Verification items for the finished model (mm, model axes). A direction names the side the tool comes from. Coordinates: 2 decimals unless noted, no trailing zeros. Order: outer loops, then holes, each group sorted by start corner. A loop starts at its lowest first (then second) coordinate and runs counter-clockwise, first axis right, second up. Notation, with made-up numbers: M 4.5,35 L 41.5,35 A15 cw 41.5,53 Z; hole C 2,-9.75 d3. An arc over 180 degrees is marked long. Return JSON: item names as keys, results as strings. Group by question number.
Q1. Section check A-A, the plane x = -34. Enter the section's corners in (y, z).
Q2. Go/stop test with flat-tipped pins: pin 1 Ø3 at (y, z) = (-21, 4) entering from -X; pin 2 Ø3 at (x, z) = (26.5, 3.5) entering from +Y; pin 3 Ø1 at (x, y) = (12, 22) entering from +Z; pin 4 Ø1.5 at (x, z) = (17, -2.5) entering from -Y. Record where each tip stops, or that it passes through.
Q3. Mould release check, pull along Y, two halves, no side actions. Record for faces 5 (the face through (-27, -23, 3)), 6 (the face through (19.772, 23.235, 3.965)), 7 (the face through (-35.11, 21.01, 0.76)), 8 (the face through (-0.8, -20, 3)): pulls with the +Y half, pulls with the -Y half, needs draft (parallel to the pull), parting line crosses it, or undercut.
Q4. Section check C-C, the plane x = 27.5. Enter the section's corners in (y, z), then the cut area to 3 significant figures.
Q5. Thickness scan on probe 1 along Y at (x, z) = (34, 0.55); probe 2 along Y at (x, z) = (-12, 2.25); probe 3 along Z at (x, y) = (-17, 8). Record the ranges inside material, lowest first.
Q6. Section check D-D, the plane z = -8. Enter the section's corners in (x, y), then the cut area to 3 significant figures.
Q7. Section check B-B, the plane y = 10. Enter the section's corners in (x, z), then the cut area to 3 significant figures.
Q8. Access from +Z, -Z, +X, -X, +Y, -Y to the whole of each face (thin tool, end or side, straight path). Record for faces 1 (the face through (-32, -7, -5)), 2 (the face through (-28, -21.3, 5.5)), 3 (the face through (-20, 22, 6.5)), 4 (the face through (27, -20, 7)).
from build123d import *

# Parameters (mm, degrees)
SKETCH_W     = 76
SKETCH_H     = 50
PAD_DEPTH    = 1.5
SKETCH001_R  = 1.5
POCKET_DEPTH = 1.501
SKETCH002_R  = 1.75
PAD001_DEPTH = 5
SKETCH003_W  = 61
SKETCH003_H  = 14
PAD002_DEPTH = 7
SKETCH004_W  = 6
SKETCH004_H  = 15
PAD003_DEPTH = 10
SKETCH005_W  = 6
SKETCH005_H  = 6
PAD004_DEPTH = 4
SKETCH006_R  = 1.75
PAD005_DEPTH = 1.5


with BuildPart() as part:
    # Sketch → Pad (new body)
    with BuildSketch(Plane.XY):
        Rectangle(SKETCH_W, SKETCH_H)
    extrude(amount=PAD_DEPTH)

    # Sketch001 (on Face6 of Pad) → Pocket (cut, through all)
    with BuildSketch(Plane.XY.offset(1.5)):
        with Locations((-34, 20)):
            Circle(SKETCH001_R)
        with Locations((34, 20)):
            Circle(SKETCH001_R)
        with Locations((-34, -20)):
            Circle(SKETCH001_R)
        with Locations((34, -20)):
            Circle(SKETCH001_R)
    extrude(amount=-POCKET_DEPTH, mode=Mode.SUBTRACT)

    # Sketch002 (on Face5 of Pocket) → Pad001 (join)
    with BuildSketch(Plane.XY.offset(1.5)):
        with Locations((-28, 21.5)):
            Circle(SKETCH002_R)
        with Locations((-20, 21.5)):
            Circle(SKETCH002_R)
        with Locations((-12, 21.5)):
            Circle(SKETCH002_R)
        with Locations((-4, 21.5)):
            Circle(SKETCH002_R)
        with Locations((4, 21.5)):
            Circle(SKETCH002_R)
        with Locations((12, 21.5)):
            Circle(SKETCH002_R)
        with Locations((20, 21.5)):
            Circle(SKETCH002_R)
        with Locations((28, 21.5)):
            Circle(SKETCH002_R)
    extrude(amount=PAD001_DEPTH)

    # Sketch003 (on Face5 of Pad001) → Pad002 (join)
    with BuildSketch(Plane.XY.offset(1.5)):
        with Locations((0, 9)):
            Rectangle(SKETCH003_W, SKETCH003_H)
    extrude(amount=PAD002_DEPTH)

    # Sketch004 (on Face4 of Pad002) → Pad003 (join)
    with BuildSketch(Plane(origin=(0, 0, 0), x_dir=(1, 0, 0), z_dir=(0, 0, -1))):
        with Locations((-35, 7.5)):
            Rectangle(SKETCH004_W, SKETCH004_H)
    extrude(amount=PAD003_DEPTH)

    # Sketch005 (on Face5 of Pad003) → Pad004 (join)
    with BuildSketch(Plane.XY.offset(1.5)):
        with Locations((-26.6, -20)):
            Rectangle(SKETCH005_W, SKETCH005_H)
        with Locations((-19, -20)):
            Rectangle(SKETCH005_W, SKETCH005_H)
        with Locations((-11.4, -20)):
            Rectangle(SKETCH005_W, SKETCH005_H)
        with Locations((-3.8, -20)):
            Rectangle(SKETCH005_W, SKETCH005_H)
        with Locations((3.8, -20)):
            Rectangle(SKETCH005_W, SKETCH005_H)
        with Locations((11.4, -20)):
            Rectangle(SKETCH005_W, SKETCH005_H)
        with Locations((19, -20)):
            Rectangle(SKETCH005_W, SKETCH005_H)
        with Locations((26.6, -20)):
            Rectangle(SKETCH005_W, SKETCH005_H)
    extrude(amount=PAD004_DEPTH)

    # Sketch006 (on Face67 of Pad004) → Pad005 (join)
    with BuildSketch(Plane.XY.offset(5.5)):
        with Locations((-26.6, -20)):
            Circle(SKETCH006_R)
        with Locations((-19, -20)):
            Circle(SKETCH006_R)
        with Locations((-11.4, -20)):
            Circle(SKETCH006_R)
        with Locations((-3.8, -20)):
            Circle(SKETCH006_R)
        with Locations((3.8, -20)):
            Circle(SKETCH006_R)
        with Locations((11.4, -20)):
            Circle(SKETCH006_R)
        with Locations((19, -20)):
            Circle(SKETCH006_R)
        with Locations((26.6, -20)):
            Circle(SKETCH006_R)
    extrude(amount=PAD005_DEPTH)


solid = part.part
Numbers:
{
 "1": {"outline": "M -25,0 L -21.5,0 L -21.5,1.5 L -25,1.5 Z; M -18.5,0 L -15,0 L -15,-10 L 0,-10 L 0,0 L 18.5,0 L 18.5,1.5 L -18.5,1.5 Z; M 21.5,0 L 25,0 L 25,1.5 L 21.5,1.5 Z"},
 "2": {"pin 1": "stops at x = -29.6", "pin 2": "stops at y = 23.25", "pin 3": "stops at z = 6.5", "pin 4": "passes through"},
 "3": {"face 5": "pulls with the -Y half", "face 6": "undercut", "face 7": "undercut", "face 8": "needs draft"},
 "4": {"outline": "M -25,0 L 25,0 L 25,1.5 L 23.18,1.5 L 23.18,6.5 L 19.82,6.5 L 19.82,1.5 L 16,1.5 L 16,8.5 L 2,8.5 L 2,1.5 L -17,1.5 L -17,5.5 L -18.5,5.5 L -18.5,7 L -21.5,7 L -21.5,5.5 L -23,5.5 L -23,1.5 L -25,1.5 Z", "area": "218 mm2"},
 "5": {"probe 1": "y = -25 to -21.5, -18.5 to 18.5, 21.5 to 25", "probe 2": "y = -23 to -17, 2 to 16, 19.75 to 23.25", "probe 3": "z = 0 to 8.5"},
 "6": {"outline": "M -38,-15 L -32,-15 L -32,0 L -38,0 Z", "area": "90.0 mm2"},
 "7": {"outline": "M -38,0 L 38,0 L 38,1.5 L 30.5,1.5 L 30.5,8.5 L -30.5,8.5 L -30.5,1.5 L -38,1.5 Z", "area": "541 mm2"},
 "8": {"face 1": "-Z, +X, +Y, -Y", "face 2": "+Z", "face 3": "+Z, +X, -X, +Y", "face 4": "+Z, +X, -X, -Y"}
}
